Part model, mm, in its own coordinate system. Round coordinates to 2 decimals unless told otherwise and drop trailing zeros. Write each loop counter-clockwise with the first axis right and the second up, starting at its lowest first coordinate (ties: lowest second). Pieces come first, ordered by that corner, then holes. Notation, with made-up numbers: M 20,-12.5 L 55,-12.5 A13 ccw 55,4.5 Z; hole C 86.25,32.25 d10. An arc over 180 degrees is marked long. Answer as a JSON object with one key per item and string values. Group by question number.
1. Band-saw the part on D-D, the plane x = 0.9. Count the separate pieces of the cut face and the enclosed holes in it, plus the area to 3 significant figures.
2. Band-saw the part on B-B, the plane y = 25.5. Write the cut outline in (x, z).
3. Drop flat-ended pins along their axis: pin 1 (1.8 mm diameter, centred on x = 3, z = -55.5, fed in from -Y); pin 2 (3 mm diameter, centred on x = 1.5, y = 84.5, fed in from -Z) (3 decimals). Give the stop position or say it passes through.
4. Band-saw the part on C-C, the plane y = 57.5. Write the cut outline in (x, z).
5. Drill centre lines: line 1 (Z direction, x = 1.25, y = 47); line 2 (Z direction, x = 5.05, y = 53.5); line 3 (Y direction, x = 3.95, z = -137). Where is each one in solid material? Low to high. Write a range as from..to.
6. Band-saw the part on A-A, the plane z = -22.5. Write the cut outline in (x, y), plus the area to 3 significant figures.
from build123d import *

# Parameters (mm, degrees)
GRUNDFORM_DEPTH          = 6
SKIZZE2_W                = 15
SKIZZE2_H                = 5.9
ZAPFENDURCHBRUCH_DEPTH   = 185.556224495
VERRUNDUNG1_R            = 10
VERRUNDUNG2_R            = 3
SKIZZE3_W                = 15
SKIZZE3_H                = 5.9
ZAPFENDURCHBRUCH_2_DEPTH = 185.556224495


with BuildPart() as part:
    # Skizze1 → Grundform (new body)
    with BuildSketch(Plane(origin=(0, 0, 0), x_dir=(0, 0, -1), z_dir=(1, 0, 0))):
        Polygon((0, 0), (20, 0), (30, 30), (70, 30), (80, 0), (155, 0), (155, 60), (70, 100), (0, 100), align=None)
    extrude(amount=GRUNDFORM_DEPTH)

    # Skizze2 → Zapfendurchbruch (cut, through all)
    with BuildSketch(Plane(origin=(6, 0, 0), x_dir=(0, 0, -1), z_dir=(1, 0, 0))):
        with Locations((97.5, 46)):
            Rectangle(SKIZZE2_W, SKIZZE2_H)
        with Locations((132.5, 46)):
            Rectangle(SKIZZE2_W, SKIZZE2_H)
        with Locations((132.5, 14)):
            Rectangle(SKIZZE2_W, SKIZZE2_H)
        with Locations((97.5, 14)):
            Rectangle(SKIZZE2_W, SKIZZE2_H)
        with Locations((57.5, 84)):
            Rectangle(SKIZZE2_W, SKIZZE2_H)
        with Locations((22.5, 84)):
            Rectangle(SKIZZE2_W, SKIZZE2_H)
        with Locations((22.5, 52)):
            Rectangle(SKIZZE2_W, SKIZZE2_H)
        with Locations((57.5, 52)):
            Rectangle(SKIZZE2_W, SKIZZE2_H)
    extrude(amount=-ZAPFENDURCHBRUCH_DEPTH, mode=Mode.SUBTRACT)

    # Verrundung1
    verrundung1_edges = [part.edges().sort_by_distance(p)[0] for p in [
        (3, 100, 0),
        (3, 100, -70),
        (3, 60, -155),
    ]]
    fillet(verrundung1_edges, radius=VERRUNDUNG1_R)

    # Verrundung2
    verrundung2_edges = [part.edges().sort_by_distance(p)[0] for p in [
        (3, 0, -155),
        (3, 0, -80),
        (3, 30, -70),
        (3, 30, -30),
        (3, 0, -20),
        (3, 0, 0),
    ]]
    fillet(verrundung2_edges, radius=VERRUNDUNG2_R)

    # Skizze3 → Zapfendurchbruch 2 (cut, through all)
    with BuildSketch(Plane.ZY):
        with Locations((-132.5, 19.9)):
            Rectangle(SKIZZE3_W, SKIZZE3_H)
        with Locations((-97.5, 19.9)):
            Rectangle(SKIZZE3_W, SKIZZE3_H)
        with Locations((-57.5, 57.9)):
            Rectangle(SKIZZE3_W, SKIZZE3_H)
        with Locations((-22.5, 57.9)):
            Rectangle(SKIZZE3_W, SKIZZE3_H)
    extrude(amount=-ZAPFENDURCHBRUCH_2_DEPTH, mode=Mode.SUBTRACT)


solid = part.part
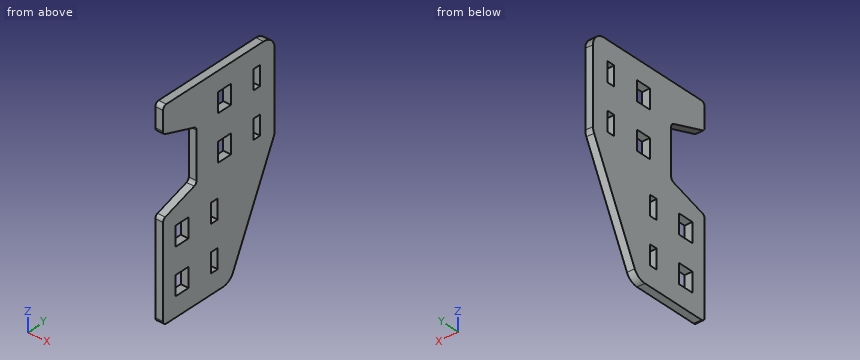
Worked answers:
{
 "1": {"separate pieces": "1", "enclosed holes": "8", "area": "11,200 mm^2"},
 "2": {"outline": "M 0,-155 L 6,-155 L 6,-71.5 L 0,-71.5 Z; M 0,-28.5 L 6,-28.5 L 6,0 L 0,0 Z"},
 "3": {"pin 1": "stops at y = 30", "pin 2": "stops at z = -106.125"},
 "4": {"outline": "M 0,-154.23 L 6,-154.23 L 6,-65 L 0,-65 Z; M 0,-50 L 6,-50 L 6,-30 L 0,-30 Z; M 0,-15 L 6,-15 L 6,0 L 0,0 Z"},
 "5": {"line 1": "z = -155..-140, -125..-105, -90..0", "line 2": "z = -155..-65, -50..-30, -15..0", "line 3": "y = 0..11.05, 22.85..43.05, 48.95..68.47"},
 "6": {"outline": "M 0,7.5 L 6,7.5 L 6,49.05 L 0,49.05 Z; M 0,60.85 L 6,60.85 L 6,81.05 L 0,81.05 Z; M 0,86.95 L 6,86.95 L 6,100 L 0,100 Z", "area": "449 mm^2"}
}
